Geometry: final body of the model. Coordinates: model frame, mm. Give positions to 0.01 mm unless a question says otherwise; leave off trailing zeros. Order: outer loops, then holes, each group sorted by start corner. A loop starts at its lowest first (then second) coordinate and runs counter-clockwise, first axis right, second up. Notation, with made-up numbers: (-4.75, 47) - (17.25, 47) arc R28 ccw to (17.25, 82) - close; hole circle Ø1 at (-6.5, -5). An arc over 180 degrees is marked (long way). One line per item, written item: value.
```python
from build123d import *

# Parameters (mm, degrees)
MODEL_R             = 3.2639
MODEL_R_2           = 15.24
BOSS_EXTRUDE1_DEPTH = 3.175
SKETCH1_R           = 2.049665702
CUT_EXTRUDE1_DEPTH  = 4.175


with BuildPart() as part:
    # Model → Boss-Extrude1 (new body)
    with BuildSketch(Plane.XY):
        Polygon((52.780663663, 19.962036807), (84.57472724, 19.962036807), (84.57472724, -20.117524571), (52.800441441, -20.117524571), (51.022441441, -20.110851742), (13.987013039, -20.110851742), (-17.005125185, -20.115733226), (-16.985347623, 19.94996289), (14.006790818, 19.955743846), (51.002663663, 19.962109065), align=None)
        with Locations((17.703224546, 14.890349751)):
            Circle(MODEL_R, mode=Mode.SUBTRACT)
        with Locations((47.70316443, 14.892992778)):
            Circle(MODEL_R, mode=Mode.SUBTRACT)
        with Locations((17.469307033, -15.107191493)):
            Circle(MODEL_R, mode=Mode.SUBTRACT)
        with Locations((47.46924701, -15.106035251)):
            Circle(MODEL_R, mode=Mode.SUBTRACT)
        with Locations((32.50472724, -0.168751446)):
            Circle(MODEL_R_2, mode=Mode.SUBTRACT)
    extrude(amount=-BOSS_EXTRUDE1_DEPTH)

    # Sketch1 → Cut-Extrude1 (cut, through all)
    with BuildSketch(Plane(origin=(0, 0, -3.175), x_dir=(-1, 0, 0), z_dir=(0, 0, -1))):
        with Locations((1.835627279, -0.168751446)):
            Circle(SKETCH1_R)
        with Locations((-66.84508176, -0.168751446)):
            Circle(SKETCH1_R)
    extrude(amount=-CUT_EXTRUDE1_DEPTH, mode=Mode.SUBTRACT)


solid = part.part
```
1) Section D-D, the plane y = 5.5. Return loops of the section in (x, z) (3 decimals), then the cut area to 3 significant figures.
Answers below:
outline: (-16.992, -3.175) - (18.358, -3.175) - (18.358, 0) - (-16.992, 0) - close; (46.651, -3.175) - (84.575, -3.175) - (84.575, 0) - (46.651, 0) - close
area: 233 mm^2
2) Section B-B, the plane y = 17. Return loops of the section in (x, z) (3 decimals), then the cut area to 3 significant figures.
Answers below:
outline: (-16.987, -3.175) - (15.213, -3.175) - (15.213, 0) - (-16.987, 0) - close; (20.194, -3.175) - (45.21, -3.175) - (45.21, 0) - (20.194, 0) - close; (50.196, -3.175) - (84.575, -3.175) - (84.575, 0) - (50.196, 0) - close
area: 291 mm^2
3) Section C-C, the plane z = -1.25. Return loops of the section in (x, y), then the cut area to 3 significant figures.
Answers below:
outline: (-17.01, -20.12) - (13.99, -20.11) - (51.02, -20.11) - (52.8, -20.12) - (84.57, -20.12) - (84.57, 19.96) - (52.78, 19.96) - (51, 19.96) - (14.01, 19.96) - (-16.99, 19.95) - close; hole circle Ø4.1 at (-1.84, -0.17); hole circle Ø6.53 at (17.47, -15.11); hole circle Ø6.53 at (17.7, 14.89); hole circle Ø30.48 at (32.5, -0.17); hole circle Ø6.53 at (47.47, -15.11); hole circle Ø6.53 at (47.7, 14.89); hole circle Ø4.1 at (66.85, -0.17)
area: 3,180 mm^2
4) Section A-A, the plane x = 18.5. Return loops of the section in (y, z) (1 decimal), then the cut area to 3 significant figures.
Answers below:
outline: (-20.1, -3.2) - (-18.2, -3.2) - (-18.2, 0) - (-20.1, 0) - close; (-12, -3.2) - (-6.2, -3.2) - (-6.2, 0) - (-12, 0) - close; (5.8, -3.2) - (11.7, -3.2) - (11.7, 0) - (5.8, 0) - close; (18.1, -3.2) - (20, -3.2) - (20, 0) - (18.1, 0) - close
area: 49.3 mm^2
5) First-contact query: pin 1 (1 mm diameter, centred on x = 26.5, z = -2.5, fed in from -Y); pin 2 (1 mm diameter, centred on x = 67, y = 0, fed in from +Z); pin 3 (8.5 mm diameter, centred on x = 47.47, y = -15.11, fed in from -Z) (3 decimals); pin 4 (1.5 mm diameter, centred on y = 8, z = -1, fed in from -X). Flat tips, straight axial feed; report the tip coordinate or a pass-through.
Answers below:
pin 1: y = -20.11
pin 2: through
pin 3: z = -3.175
pin 4: x = -16.99
6) Material intervals for line 1 along X through (y, z) = (-0.5, -2.6); line 2 along Y through (x, z) = (15, -1.5); line 3 along X through (y, z) = (-18, -2.5), sorted ascending.
Answers below:
line 1: -17 to -3.86, 0.19 to 17.27, 47.74 to 64.82, 68.87 to 84.57
line 2: -20.11 to -17.24, -12.97 to 13.06, 16.72 to 19.96
line 3: -17 to 15.96, 18.98 to 45.96, 48.98 to 84.57
7) Mould query, pull axis X, two halves, no side actions, for faces 1 (the face through (16.8, -18.3, -1.6)), 2 (the face through (84.575, 0, -2)), 3 (the face through (46, 9, -3.175)). Classes: released by +X, released by -X, zero draft, split by the parting line, or undercut.
Answers below:
face 1: undercut
face 2: released by +X
face 3: zero draft
